Verification items for the finished model (mm, model axes). A direction names the side the tool comes from. Give positions to 0.01 mm unless a question says otherwise; leave off trailing zeros. Write each loop counter-clockwise with the first axis right and the second up, starting at its lowest first coordinate (ties: lowest second). Pieces come first, ordered by that corner, then holes.
from build123d import *

# Parameters (mm, degrees)
F0_W     = 12.7
F0_H     = 24.60625
F0_H_2   = 39.6875
F1_DEPTH = 12.7
F2_DEPTH = 3.175
F3_DEPTH = 6.35


with BuildPart() as f1:
    # F0 (on Front) → F1 (new body)
    with BuildSketch(Plane.XZ):
        with BuildLine():
            Line((-196.85, 97.63125), (-196.85, 122.2375))
            ThreePointArc((-196.85, 122.2375), (-205.830256, 118.517756), (-209.55, 109.5375))
            Line((-209.55, 109.5375), (-209.55, -109.5375))
            ThreePointArc((-209.55, -109.5375), (-205.830256, -118.517756), (-196.85, -122.2375))
            Line((-196.85, -122.2375), (-196.85, -97.63125))
            Line((-196.85, -97.63125), (-196.85, -19.84375))
            Line((-196.85, -19.84375), (-196.85, 19.84375))
            Line((-196.85, 19.84375), (-196.85, 97.63125))
        make_face()
        with Locations((-190.5, 109.934375)):
            Rectangle(F0_W, F0_H)
        with Locations((-190.5, 0)):
            Rectangle(F0_W, F0_H_2)
        with Locations((-190.5, -109.934375)):
            Rectangle(F0_W, F0_H)
        with BuildLine():
            Line((-180.975, 122.2375), (-184.15, 122.2375))
            Line((-184.15, 122.2375), (-184.15, 97.63125))
            Line((-184.15, 97.63125), (-184.15, 19.84375))
            Line((-184.15, 19.84375), (-184.15, -19.84375))
            Line((-184.15, -19.84375), (-184.15, -97.63125))
            Line((-184.15, -97.63125), (-184.15, -122.2375))
            Line((-184.15, -122.2375), (184.15, -122.2375))
            Line((184.15, -122.2375), (184.15, -97.63125))
            Line((184.15, -97.63125), (184.15, -19.84375))
            Line((184.15, -19.84375), (184.15, 19.84375))
            Line((184.15, 19.84375), (184.15, 97.63125))
            Line((184.15, 97.63125), (184.15, 122.2375))
            Line((184.15, 122.2375), (180.975, 122.2375))
            ThreePointArc((180.975, 122.2375), (178.729936, 121.307564), (177.8, 119.0625))
            Line((177.8, 119.0625), (177.8, 109.5375))
            ThreePointArc((177.8, 109.5375), (176.870064, 107.292436), (174.625, 106.3625))
            Line((174.625, 106.3625), (-174.625, 106.3625))
            ThreePointArc((-174.625, 106.3625), (-176.870064, 107.292436), (-177.8, 109.5375))
            Line((-177.8, 109.5375), (-177.8, 119.0625))
            ThreePointArc((-177.8, 119.0625), (-178.729936, 121.307564), (-180.975, 122.2375))
        make_face()
        with Locations((190.5, -109.934375)):
            Rectangle(F0_W, F0_H)
        with BuildLine():
            ThreePointArc((209.55, 109.5375), (205.830256, 118.517756), (196.85, 122.2375))
            Line((196.85, 122.2375), (196.85, 97.63125))
            Line((196.85, 97.63125), (196.85, 19.84375))
            Line((196.85, 19.84375), (196.85, -19.84375))
            Line((196.85, -19.84375), (196.85, -97.63125))
            Line((196.85, -97.63125), (196.85, -122.2375))
            ThreePointArc((196.85, -122.2375), (205.830256, -118.517756), (209.55, -109.5375))
            Line((209.55, -109.5375), (209.55, 109.5375))
        make_face()
        with Locations((190.5, 0)):
            Rectangle(F0_W, F0_H_2)
        with Locations((190.5, 109.934375)):
            Rectangle(F0_W, F0_H)
        with BuildLine():
            Line((180.975, 122.2375), (-180.975, 122.2375))
            ThreePointArc((-180.975, 122.2375), (-178.729936, 121.307564), (-177.8, 119.0625))
            Line((-177.8, 119.0625), (-177.8, 109.5375))
            ThreePointArc((-177.8, 109.5375), (-176.870064, 107.292436), (-174.625, 106.3625))
            Line((-174.625, 106.3625), (174.625, 106.3625))
            ThreePointArc((174.625, 106.3625), (176.870064, 107.292436), (177.8, 109.5375))
            Line((177.8, 109.5375), (177.8, 119.0625))
            ThreePointArc((177.8, 119.0625), (178.729936, 121.307564), (180.975, 122.2375))
        make_face()
    extrude(amount=-F1_DEPTH)

    # F0 (on Front) → F2 (cut)
    with BuildSketch(Plane.XZ):
        with Locations((-190.5, -109.934375)):
            Rectangle(F0_W, F0_H)
        with Locations((-190.5, 0)):
            Rectangle(F0_W, F0_H_2)
        with Locations((190.5, -109.934375)):
            Rectangle(F0_W, F0_H)
        with Locations((190.5, 0)):
            Rectangle(F0_W, F0_H_2)
        with Locations((190.5, 109.934375)):
            Rectangle(F0_W, F0_H)
        with Locations((-190.5, 109.934375)):
            Rectangle(F0_W, F0_H)
    extrude(amount=-F2_DEPTH, mode=Mode.SUBTRACT)

    # F0 (on Front) → F3 (cut)
    with BuildSketch(Plane.XZ):
        with BuildLine():
            Line((180.975, 122.2375), (-180.975, 122.2375))
            ThreePointArc((-180.975, 122.2375), (-178.729936, 121.307564), (-177.8, 119.0625))
            Line((-177.8, 119.0625), (-177.8, 109.5375))
            ThreePointArc((-177.8, 109.5375), (-176.870064, 107.292436), (-174.625, 106.3625))
            Line((-174.625, 106.3625), (174.625, 106.3625))
            ThreePointArc((174.625, 106.3625), (176.870064, 107.292436), (177.8, 109.5375))
            Line((177.8, 109.5375), (177.8, 119.0625))
            ThreePointArc((177.8, 119.0625), (178.729936, 121.307564), (180.975, 122.2375))
        make_face()
    extrude(amount=-F3_DEPTH, mode=Mode.SUBTRACT)


solid = f1.part
Item 1: Sectioned sample at D-D on z = -105. Record the cut outline in (x, y) (3 decimals), then the cut area to 3 significant figures.
Answer key:
outline: (-209.55, 0) - (-196.85, 0) - (-196.85, 3.175) - (-184.15, 3.175) - (-184.15, 0) - (184.15, 0) - (184.15, 3.175) - (196.85, 3.175) - (196.85, 0) - (209.55, 0) - (209.55, 12.7) - (-209.55, 12.7) - close
area: 5,240 mm2
Item 2: Sectioned sample at B-B on z = 93. Record the cut outline in (x, y).
Answer key:
outline: (-209.55, 0) - (-196.85, 0) - (-196.85, 12.7) - (-209.55, 12.7) - close; (-184.15, 0) - (184.15, 0) - (184.15, 12.7) - (-184.15, 12.7) - close; (196.85, 0) - (209.55, 0) - (209.55, 12.7) - (196.85, 12.7) - close
Item 3: Set-up check for faces 1 (the face through (203, 0, 2)), 2 (the face through (190, 8, -19.844)), 3 (the face through (190, 3.175, 0)): record each of +Z, -Z, +X, -X, +Y, -Y from which the full face is reachable in a straight line by a thin tool's end or side.
Answer key:
face 1: +Z, -Z, +X, -X, -Y
face 2: +Y, -Y
face 3: +Z, -Z, -Y
Item 4: Sectioned sample at C-C on x = 10. Record the cut outline in (y, z).
Answer key:
outline: (0, -122.24) - (12.7, -122.24) - (12.7, 122.24) - (6.35, 122.24) - (6.35, 106.36) - (0, 106.36) - close
Item 5: Sectioned sample at A-A on y = 8.5. Record the cut outline in (x, z), then the cut area to 3 significant figures.
Answer key:
outline: (-209.55, -109.54) arc R12.7 ccw to (-196.85, -122.24) - (196.85, -122.24) arc R12.7 ccw to (209.55, -109.54) - (209.55, 109.54) arc R12.7 ccw to (196.85, 122.24) - (-196.85, 122.24) arc R12.7 ccw to (-209.55, 109.54) - close; hole (-196.85, -97.63) - (-184.15, -97.63) - (-184.15, -19.84) - (-196.85, -19.84) - close; hole (-196.85, 19.84) - (-184.15, 19.84) - (-184.15, 97.63) - (-196.85, 97.63) - close; hole (184.15, -97.63) - (196.85, -97.63) - (196.85, -19.84) - (184.15, -19.84) - close; hole (184.15, 19.84) - (196.85, 19.84) - (196.85, 97.63) - (184.15, 97.63) - close
area: 98,400 mm2
Item 6: Release check for a two-part mould opening along Z. For faces 4 (the face through (3, 9, 122.237)), 5 (the face through (-191, 3.175, 0)), 6 (the face through (-191, 8, 97.631)) record: released by +Z, released by -Z, zero draft, split by the parting line, or undercut.
Answer key:
face 4: released by +Z
face 5: zero draft
face 6: undercut
Item 7: Depth check by flat-ended pin: pin 1 (4 mm diameter, centred on x = -188.5, z = -107.5, fed in from -Y) (3 decimals); pin 2 (5 mm diameter, centred on x = 80, z = 111, fed in from -Y). Enter the tip coordinate at first touch or a pass-through.
Answer key:
pin 1: stops at y = 3.175
pin 2: stops at y = 6.35
Item 8: Scan lines: line 1 along X through (y, z) = (9.25, 28); line 2 along Z through (x, y) = (-186, 5); line 3 along Z through (x, y) = (-66, 3). Record each from-to range of solid material in increasing order.
Answer key:
line 1: x = -209.55 to -196.85, -184.15 to 184.15, 196.85 to 209.55
line 2: z = -122.24 to -97.63, -19.84 to 19.84, 97.63 to 122.24
line 3: z = -122.24 to 106.36
